Part print with two shaded views. Sizes in mm from the minimum x, y, z corner. A direction names the side the tool comes from. Give positions to 0.01 mm unless a question says otherwise; leave off trailing zeros. Order: outer loops, then holes, each group sorted by start corner. A loop starts at its lowest first (then second) coordinate and runs counter-clockwise, first axis right, second up. Notation, with made-up numbers: M 85.25,24.5 L 140.25,24.5 A19 cw 140.25,59.5 Z; hole C 66,85.25 d10. An arc over 180 degrees is marked long. Return JSON: item names as keys, results as strings.
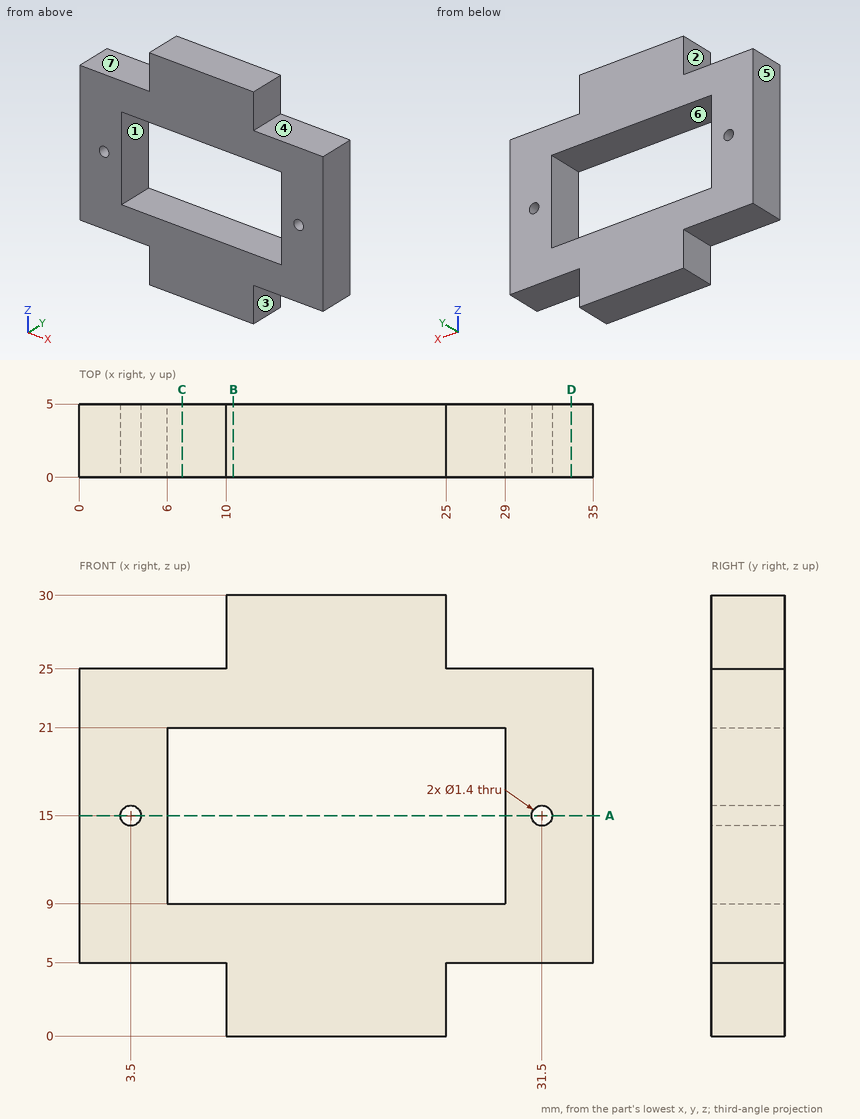
Q1. 3-axis set-ups, long thin cutter, end or side, ignore diameter. For the marked faces 1, 2, 3 and 4: which of +Z, -Z, +X, -X, +Y, -Y reach the whole face in a straight line?
Established:
{"face 1": "+Y, -Y", "face 2": "+Z, -X, +Y, -Y", "face 3": "-Z, +X, +Y, -Y", "face 4": "+Z, +X, +Y, -Y"}
Q2. Band-saw the part on D-D (x = 33.5). Give the cut face in (y, z), then the cut area to 3 significant figures.
Established:
{"outline": "M 0,5 L 5,5 L 5,25 L 0,25 Z", "area": "100 mm²"}
Q3. Probe line 1 along X through (y, z) = (3.7, 15); line 2 along Z through (x, y) = (14.5, 1.95); line 3 along Z through (x, y) = (28, 4.2). List the from-to ranges inside material, lowest first.
Established:
{"line 1": "x = 0 to 2.8, 4.2 to 6, 29 to 30.8, 32.2 to 35", "line 2": "z = 0 to 9, 21 to 30", "line 3": "z = 5 to 9, 21 to 25"}
Q4. Band-saw the part on B-B (x = 10.5). Give the cut face in (y, z), then the cut area to 3 significant figures.
Established:
{"outline": "M 0,0 L 5,0 L 5,9 L 0,9 Z; M 0,21 L 5,21 L 5,30 L 0,30 Z", "area": "90.0 mm²"}
Q5. Band-saw the part on A-A (z = 15). Give the cut face in (x, y).
Established:
{"outline": "M 0,0 L 2.8,0 L 2.8,5 L 0,5 Z; M 4.2,0 L 6,0 L 6,5 L 4.2,5 Z; M 29,0 L 30.8,0 L 30.8,5 L 29,5 Z; M 32.2,0 L 35,0 L 35,5 L 32.2,5 Z"}
Q6. Band-saw the part on C-C (x = 7). Give the cut face in (y, z).
Established:
{"outline": "M 0,5 L 5,5 L 5,9 L 0,9 Z; M 0,21 L 5,21 L 5,25 L 0,25 Z"}
Q7. Two-plate mould, pull along X, no slides. Class the marked faces 5, 6 and 7: +X half, -X half, draft (parallel to the pull), parting line (faces both ways), or undercut.
Established:
{"face 5": "-X half", "face 6": "undercut", "face 7": "draft"}
Q8. Pin check, flat tips, straight feed: pin 1 (2 mm diameter, centred on x = 31.5, z = 15, fed in from +Y); pin 2 (1.5 mm diameter, centred on x = 3, y = 2, fed in from -Z); pin 3 (2.5 mm diameter, centred on y = 3.5, z = 2, fed in from -X); pin 4 (2.5 mm diameter, centred on x = 3, y = 1.5, fed in from +Z). Stop position of each tip, or through.
Established:
{"pin 1": "stops at y = 5", "pin 2": "stops at z = 5", "pin 3": "stops at x = 10", "pin 4": "stops at z = 25"}
